from build123d import *

# Parameters (mm, degrees)
ESQUISSE1_R      = 2.5
EXTRUSION1_DEPTH = 30
ESQUISSE3_W      = 25
ESQUISSE3_H      = 24
EXTRUSION2_DEPTH = 105.777068413


with BuildPart() as part:
    # Esquisse1 → Extrusion1 (new body)
    with BuildSketch(Plane(origin=(0, 0, 0), x_dir=(1, 0, 0), z_dir=(0, 1, 0))):
        with BuildLine():
            Line((0, 0), (0, 50))
            Line((0, 50), (3, 50))
            Line((3, 50), (3, 0))
            ThreePointArc((3, 0), (9.404287474, -35.029045403), (27.788566098, -65.526048852))
            Line((27.788566098, -65.526048852), (47.644944538, -88.014362156))
            Line((47.644944538, -88.014362156), (50.26858109, -85.697784671))
            Line((50.26858109, -85.697784671), (56.887373903, -93.193889106))
            Line((56.887373903, -93.193889106), (49.391269469, -99.812681919))
            Line((49.391269469, -99.812681919), (42.772476656, -92.316577485))
            Line((42.772476656, -92.316577485), (45.396113208, -90))
            Line((45.396113208, -90), (25.539734768, -67.511686696))
            ThreePointArc((25.539734768, -67.511686696), (6.598356792, -36.090531627), (0, 0))
        make_face()
        with Locations((49.82992528, -92.755233295)):
            Circle(ESQUISSE1_R, mode=Mode.SUBTRACT)
    extrude(amount=EXTRUSION1_DEPTH)

    # Esquisse3 → Extrusion2 (cut, through all)
    with BuildSketch(Plane(origin=(-21.768488457, 0, 19.220798778), x_dir=(0.661879281, 0, 0.749610443), z_dir=(-0.749610443, 0, 0.661879281))):
        with Locations((95.011686696, 15)):
            Rectangle(ESQUISSE3_W, ESQUISSE3_H)
    extrude(amount=-EXTRUSION2_DEPTH, mode=Mode.SUBTRACT)


solid = part.part
The model under review builds one solid part; all positions refer to its coordinate system, in mm. A direction names the side the tool comes from. Give positions to 0.01 mm unless a question says otherwise; leave off trailing zeros. Write each loop counter-clockwise with the first axis right and the second up, starting at its lowest first coordinate (ties: lowest second). Pieces come first, ordered by that corner, then holes. Notation, with made-up numbers: M -25.75,22 L -14.75,22 A8 cw -14.75,35 Z; hole C 24.5,-18 d4. An arc over 180 degrees is marked long. One line per question, with ' | ' between items. Start each with the question number.
Item 1: We need section C-C on x = 5. Write out the cut boundary in (y, z).
Item 2: Draft analysis for pull direction Z (two halves, no side actions). For faces 4 (the cylindrical face through (50.984, 28.479, 94.973)), 5 (the flat face through (46.13, 1.48, 96.12)), 6 (the flat face through (0, 15, -25)), state which applies: released by +Z, released by -Z, zero draft, split by the parting line, or undercut.
Item 3: For faces 1 (the flat face through (48.94, 1.48, 86.87)), 2 (the flat face through (44.07, 1.48, 91.17)), 3 (the flat face through (3, 15, -25)), list the 3-axis set-ups (+Z, -Z, +X, -X, +Y, -Y) from which the entire face can be reached by the end or side of a thin tool; tool diameter is ignored.
Item 4: Wall thickness on line 1 (X direction, y = 3.5, z = -21.5); line 2 (X direction, y = 14.5, z = 77.5); line 3 (Z direction, x = 25, y = 13.75): over which ranges is each line inside the solid? List them lowest first. Write a range as from..to.
Item 5: We need section B-B on z = -28.5. Write out the cut boundary in (x, y).
Item 6: We need section A-A on y = 22.5. Write out the cut boundary in (x, z), plus the area to 3 significant figures.
Item 7: For pin 1 (5 mm diameter, centred on x = 27.5, y = 22.5, fed in from -Z); pin 2 (3 mm diameter, centred on x = 27, y = 23.5, fed in from +Z); pin 3 (9 mm diameter, centred on y = 20.5, z = -16, fed in from +X), all flat-tipped, find the tip position at first contact; note any pin that passes through.
Results found:
1) outline: M 0,19.8 L 30,19.8 L 30,31.54 L 0,31.54 Z
2) face 4: undercut | face 5: released by +Z | face 6: zero draft
3) face 1: -Z, +Y, -Y | face 2: -X, +Y, -Y | face 3: -Z, +X, +Y, -Y
4) line 1: x = 0..3 | line 2: x = 34.36..36.89 | line 3: z = 62.23..66.9
5) outline: M 0,0 L 3,0 L 3,30 L 0,30 Z
6) outline: M 0,-50 L 3,-50 L 3,0 A99 cw 27.79,65.53 L 37.72,76.77 L 35.47,78.76 L 25.54,67.51 A102 ccw 0,0 Z | area: 413 mm2
7) pin 1: stops at z = 62.23 | pin 2: stops at z = 70.86 | pin 3: stops at x = 3
